from build123d import *

# Parameters (mm, degrees)
SKETCH1_R               = 54.5
SKETCH1_R_2             = 44.5
BOSS_EXTRUDE1_DEPTH     = 20
CUT_EXTRUDE1_REACH      = 81.627
CUT_EXTRUDE1_END_RADIUS = 54.5
SKETCH2_R               = 3.175
CUT_EXTRUDE2_REACH      = 81.627
CUT_EXTRUDE2_END_RADIUS = 54.5
SKETCH2_2_R             = 3.175
SKETCH3_W               = 5
SKETCH3_H               = 9.5
BOSS_EXTRUDE2_DEPTH     = 13
CUT_EXTRUDE3_REACH      = 87.488
CUT_EXTRUDE4_REACH      = 87.392
SKETCH5_R               = 2.38125
SKETCH6_R               = 3.175
CUT_EXTRUDE5_DEPTH      = 180
SKETCH8_R               = 4.826
CUT_EXTRUDE6_DEPTH      = 5
SKETCH9_R               = 6.35
CUT_EXTRUDE7_DEPTH      = 1
SKETCH10_R              = 6.35
CUT_EXTRUDE9_DEPTH      = 1


with BuildPart() as part:
    # Sketch1 → Boss-Extrude1 (new body)
    with BuildSketch(Plane(origin=(0, 0, 0), x_dir=(1, 0, 0), z_dir=(0, 1, 0))):
        with Locations(Location((0, 0, 0), (0, 0, 270))):
            Circle(SKETCH1_R)
        with Locations(Location((0, 0, 0), (0, 0, 270))):
            Circle(SKETCH1_R_2, mode=Mode.SUBTRACT)
    extrude(amount=BOSS_EXTRUDE1_DEPTH)

    # Cut-Extrude1: up to this cylinder (the profile starts inside it)
    cut_extrude1_end = Plane(origin=(0, 10, 0), z_dir=(0, -1, 0)) * Cylinder(CUT_EXTRUDE1_END_RADIUS, 273.254, mode=Mode.PRIVATE)
    # Sketch2 → Cut-Extrude1 (cut, up to the surface)
    with BuildSketch(Plane.XY, mode=Mode.PRIVATE) as cut_extrude1_sk1:
        with Locations((0, 10)):
            Circle(SKETCH2_R)
    cut_extrude1_tool1 = extrude(cut_extrude1_sk1.sketch, amount=-CUT_EXTRUDE1_REACH, mode=Mode.PRIVATE) & cut_extrude1_end
    add(cut_extrude1_tool1.solids().sort_by_distance((0, 10, 0))[0], mode=Mode.SUBTRACT)

    # Cut-Extrude2: up to this cylinder (the profile starts inside it)
    cut_extrude2_end = Plane(origin=(0, 10, 0), z_dir=(0, -1, 0)) * Cylinder(CUT_EXTRUDE2_END_RADIUS, 273.254, mode=Mode.PRIVATE)
    # Sketch2_2 → Cut-Extrude2 (cut, up to the surface)
    with BuildSketch(Plane.XY, mode=Mode.PRIVATE) as cut_extrude2_sk1:
        with Locations((0, 10)):
            Circle(SKETCH2_2_R)
    cut_extrude2_tool1 = extrude(cut_extrude2_sk1.sketch, amount=CUT_EXTRUDE2_REACH, mode=Mode.PRIVATE) & cut_extrude2_end
    add(cut_extrude2_tool1.solids().sort_by_distance((0, 10, 0))[0], mode=Mode.SUBTRACT)

    # Sketch3 → Boss-Extrude2 (add)
    with BuildSketch(Plane(origin=(0, 20, 0), x_dir=(1, 0, 0), z_dir=(0, 1, 0))):
        with Locations((0, -49.5)):
            Rectangle(SKETCH3_W, SKETCH3_H)
    boss_extrude2 = extrude(amount=BOSS_EXTRUDE2_DEPTH)

    # Sketch4 → Cut-Extrude3 (cut, up to next)
    with BuildSketch(Plane(origin=(2.5, 0, 0), x_dir=(0, 0, -1), z_dir=(1, 0, 0)), mode=Mode.PRIVATE) as cut_extrude3_sk1:
        with BuildLine():
            Line((-54.25, 28), (-54.25, 33))
            Line((-54.25, 33), (-44.75, 33))
            Line((-44.75, 33), (-44.75, 28))
            ThreePointArc((-44.75, 28), (-49.5, 32.75), (-54.25, 28))
        make_face()
    cut_extrude3_tool1 = extrude(cut_extrude3_sk1.sketch, amount=-CUT_EXTRUDE3_REACH, mode=Mode.PRIVATE) & part.part
    cut_extrude3 = cut_extrude3_tool1.solids().sort_by_distance((2.5, 32.857355, 49.5))[0]
    add(cut_extrude3, mode=Mode.SUBTRACT)

    # Sketch5 → Cut-Extrude4 (cut, up to next)
    with BuildSketch(Plane(origin=(2.5, 0, 0), x_dir=(0, 0, -1), z_dir=(1, 0, 0)), mode=Mode.PRIVATE) as cut_extrude4_sk1:
        with Locations((-49.5, 28)):
            Circle(SKETCH5_R)
    cut_extrude4_tool1 = extrude(cut_extrude4_sk1.sketch, amount=-CUT_EXTRUDE4_REACH, mode=Mode.PRIVATE) & part.part
    cut_extrude4 = cut_extrude4_tool1.solids().sort_by_distance((2.5, 28, 49.5))[0]
    add(cut_extrude4, mode=Mode.SUBTRACT)

    # Mirror1: Boss-Extrude2, Cut-Extrude3, Cut-Extrude4 across plane
    add(boss_extrude2.mirror(Plane.XY))
    add(cut_extrude3.mirror(Plane.XY), mode=Mode.SUBTRACT)
    add(cut_extrude4.mirror(Plane.XY), mode=Mode.SUBTRACT)

    # Sketch6 → Cut-Extrude5 (cut)
    with BuildSketch(Plane(origin=(54.5, 0, 0), x_dir=(0, 0, -1), z_dir=(1, 0, 0))):
        with Locations((0, 10)):
            Circle(SKETCH6_R)
    extrude(amount=-CUT_EXTRUDE5_DEPTH, mode=Mode.SUBTRACT)

    # Sketch8 → Cut-Extrude6 (cut)
    with BuildSketch(Plane.XY.offset(54.5)):
        with Locations((0, 10)):
            Circle(SKETCH8_R)
    cut_extrude6 = extrude(amount=-CUT_EXTRUDE6_DEPTH, mode=Mode.SUBTRACT)

    # Mirror2: Cut-Extrude6 across plane
    add(cut_extrude6.mirror(Plane.XY), mode=Mode.SUBTRACT)

    # Sketch9 → Cut-Extrude7 (cut)
    with BuildSketch(Plane(origin=(54.5, 0, 0), x_dir=(0, 0, -1), z_dir=(1, 0, 0))):
        with Locations((0, 10)):
            Circle(SKETCH9_R)
    cut_extrude7 = extrude(amount=-CUT_EXTRUDE7_DEPTH, mode=Mode.SUBTRACT)

    # Mirror3: Cut-Extrude7 across plane
    add(cut_extrude7.mirror(Plane(origin=(0, 0, 0), x_dir=(0, 0, 1), z_dir=(1, 0, 0))), mode=Mode.SUBTRACT)

    # Sketch10 → Cut-Extrude9 (cut, symmetric)
    with BuildSketch(Plane.XY.offset(44.5)):
        with Locations(Location((0, 10, 0), (0, 0, 180))):
            Circle(SKETCH10_R)
    cut_extrude9 = extrude(amount=CUT_EXTRUDE9_DEPTH, both=True, mode=Mode.SUBTRACT)

    # Mirror4: Cut-Extrude9 across plane
    add(cut_extrude9.mirror(Plane.XY), mode=Mode.SUBTRACT)


solid = part.part
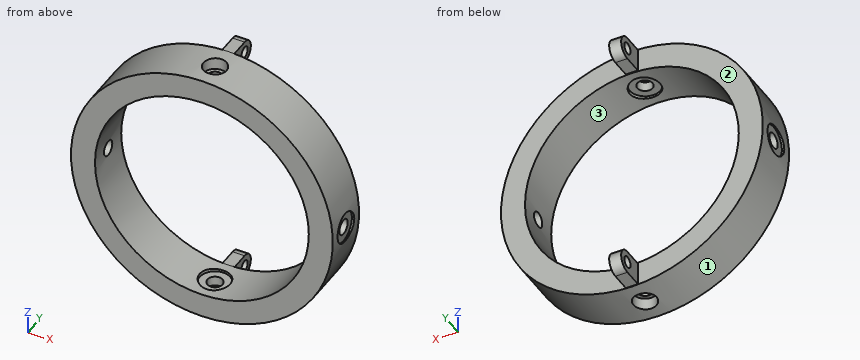
Can you work these out from the model? Positions are in its coordinate system, mm. Face numbers are marked on the shaded views. Give positions to 0.01 mm unless a question says otherwise; leave off trailing zeros. Order: outer loops, then holes, each group sorted by start corner. A loop starts at its lowest first (then second) coordinate and runs counter-clockwise, first axis right, second up. Notation, with made-up numbers: M 89.25,35.25 L 146.25,35.25 A23 ccw 146.25,70.25 Z; hole C 81.25,-30 d7. An arc over 180 degrees is marked long. One line per item, written item: value.
Item 1: If we section it at B-B on x = 17: Write out the boundary of the cut face in (y, z), and give its area (3 significant figures).
Verdict:
outline: M 0,-51.78 L 20,-51.78 L 20,-41.12 L 0,-41.12 Z; M 0,41.12 L 20,41.12 L 20,51.78 L 0,51.78 Z
area: 426 mm2
Item 2: For pin 1 (3 mm diameter, centred on x = 0, y = 12, fed in from +Z); pin 2 (6 mm diameter, centred on y = 6.5, z = -2.5, fed in from -X); pin 3 (5 mm diameter, centred on y = 24.5, z = 47.5, fed in from -X); pin 4 (10 mm diameter, centred on x = 0, y = 10, fed in from +Z), each with a flat end and sliding along its axis, tell me the tip position at first contact or that it passes through.
Verdict:
pin 1: z = 49.5
pin 2: x = -54.49
pin 3: x = -2.5
pin 4: z = 54.5
Item 3: If we mould it in two halves opening along X, with no side actions, what happens to the marked faces 1, 2 and 3? For each: pulls with the +X half, pulls with the -X half, needs draft (parallel to the pull), parting line crosses it, or undercut.
Verdict:
face 1: parting line crosses it
face 2: needs draft
face 3: undercut
Item 4: Please list where these lines run through material, in increasing order: line 1 (Z direction, x = -10.5, y = 3); line 2 (X direction, y = 4, z = -33); line 3 (Z direction, x = 0, y = 6).
Verdict:
line 1: -53.48 to -43.24, 43.24 to 53.48
line 2: -43.37 to -29.85, 29.85 to 43.37
line 3: -49.5 to -45.5, 45.5 to 49.5
Item 5: If we section it at C-C on x = 0: State how many separate pieces and enclosed holes the cut face has, and give its area (3 significant figures).
Verdict:
separate pieces: 4
enclosed holes: 2
area: 415 mm2
Item 6: If we section it at A-A on z = 0: Write out the boundary of the cut face in (x, y) (3 decimals), and give its area (3 significant figures).
Verdict:
outline: M -54.5,0 L -44.5,0 L -44.5,6.825 L -53.5,6.825 L -53.5,3.65 L -54.5,3.65 Z; M -54.5,16.35 L -53.5,16.35 L -53.5,13.175 L -44.5,13.175 L -44.5,20 L -54.5,20 Z; M 44.5,0 L 54.5,0 L 54.5,3.65 L 53.5,3.65 L 53.5,6.825 L 44.5,6.825 Z; M 44.5,13.175 L 53.5,13.175 L 53.5,16.35 L 54.5,16.35 L 54.5,20 L 44.5,20 Z
area: 260 mm2
Item 7: If we section it at D-D on z = 36.5: Write out the boundary of the cut face in (x, y), and give its area (3 significant figures).
Verdict:
outline: M -40.47,0 L -25.46,0 L -25.46,20 L -40.47,20 Z; M 25.46,0 L 40.47,0 L 40.47,20 L 25.46,20 Z
area: 601 mm2
